```python
from build123d import *

# Parameters (mm, degrees)
F1_DEPTH = 10
F2_R     = 3.5
F3_SIZE  = 1
F4_R     = 1


# Not quite as in the source:
# - a feature names something its author has since deleted; it is built from what else it names


with BuildPart() as f1:
    # F0 (on Top) → F1 (new body)
    with BuildSketch(Plane.XY):
        with BuildLine():
            ThreePointArc((-44.3848475016, -14.7620242305), (-53.4374201274, 3.0310367894), (-39.6333784075, 17.4529133594))
            Line((-39.6333784075, 17.4529133594), (-39.6333784075, 67.7640176489))
            ThreePointArc((-39.6333784075, 67.7640176489), (-36.3720424684, 71.025353588), (-33.1107065292, 67.7640176489))
            Line((-33.1107065292, 67.7640176489), (-33.1107065292, 17.4529133594))
            ThreePointArc((-33.1107065292, 17.4529133594), (-19.3066648093, 3.0310367894), (-28.3592374351, -14.7620242305))
            Line((-28.3592374351, -14.7620242305), (-22.5229276093, -20.2994880054))
            ThreePointArc((-22.5229276093, -20.2994880054), (-11.4323530197, 2.249497469), (-25.5391483675, 23.0450718941))
            Line((-25.5391483675, 23.0450718941), (-25.5391483675, 67.7640176489))
            ThreePointArc((-25.5391483675, 67.7640176489), (-36.3720424684, 78.5969117497), (-47.2049365692, 67.7640176489))
            Line((-47.2049365692, 67.7640176489), (-47.2049365692, 23.0450718941))
            ThreePointArc((-47.2049365692, 23.0450718941), (-61.311731917, 2.249497469), (-50.2211573274, -20.2994880054))
            Line((-50.2211573274, -20.2994880054), (-44.3848475016, -14.7620242305))
        make_face()
    extrude(amount=F1_DEPTH)

    # F2
    f2_edges = [f1.edges().sort_by_distance(p)[0] for p in [
        (-50.221157, -20.299488, 5),
        (-44.384848, -14.762024, 5),
        (-28.359237, -14.762024, 5),
        (-22.522928, -20.299488, 5),
    ]]
    fillet(f2_edges, radius=F2_R)

    # F3
    f3_edges = [f1.edges().sort_by_distance(p)[0] for p in [
        (-53.038502, 4.962794, 10),
        (-61.149218, 3.844419, 10),
        (-47.204937, 45.404545, 10),
        (-39.633378, 42.608466, 10),
        (-36.372042, 78.596912, 10),
        (-36.372042, 71.025354, 10),
        (-33.110707, 42.608466, 10),
        (-25.539148, 45.404545, 10),
        (-19.705582, 4.962794, 10),
        (-11.594867, 3.844419, 0),
        (-25.539148, 45.404545, 0),
        (-39.633378, 42.608466, 0),
        (-53.038502, 4.962794, 0),
    ]]
    chamfer(f3_edges, length=F3_SIZE)

    # F4
    f4_edges = [f1.edges().sort_by_distance(p)[0] for p in [
        (-39.633378, 17.452913, 5),
        (-33.110707, 17.452913, 5),
    ]]
    fillet(f4_edges, radius=F4_R)


solid = f1.part
```
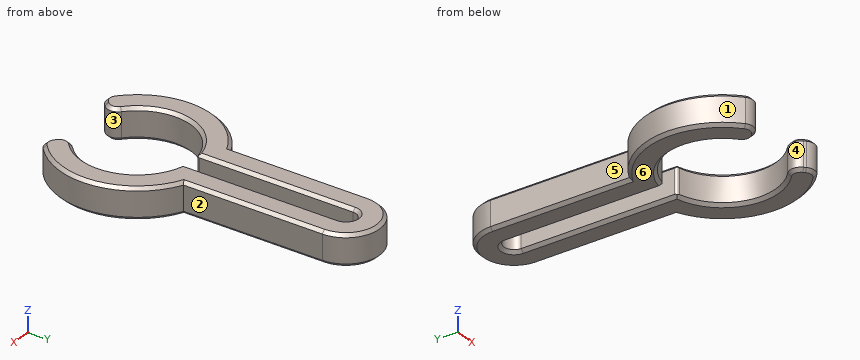
Could you check a few things on this model? Use its own coordinates, in mm. Face numbers are marked on the shaded views. A direction names the side the tool comes from. Give positions to 0.01 mm unless a question says otherwise; leave off trailing zeros. Loops run counter-clockwise (first coordinate to the right, second up) from the corner with the lowest first, then second, coordinate; pieces in that order, holes last. Notation, with made-up numbers: (79.25, 7) - (125.25, 7) arc R11 ccw to (125.25, 18) - close; hole circle Ø10 at (43, -2.75). An arc over 180 degrees is marked (long way). Answer in a Markdown table with one row per item. Add a question column.
Q1. Which directions (+Z, -Z, +X, -X, +Y, -Y) give clear straight access to the entire face, cutting with the end or side of a thin tool? Please do the marked faces 1, 2 and 3.
Q2. For pin 1 (6 mm diameter, centred on y = 4.5, z = 5.5, fed in from +X); pin 2 (4 mm diameter, centred on y = 54, z = 6.5, fed in from -X); pin 3 (4 mm diameter, centred on y = 50.5, z = 6, fed in from +X), each with a flat end and sliding along its axis, tell me the tip position at first contact or that it passes through.
Q3. Please list where these lines run through material, in increasing order: L1, parallel to X at y = 52, z = 7; L2, parallel to Y at x = -51, z = 4.75; L3, parallel to Y at x = -50.5, z = 2.25. Write a range as from..to.
Q4. We'd pull the mould along X, two halves only. Please class the marked faces 4, 5 and 6: +X half, -X half, draft (parallel to the pull), parting line (faces both ways), or undercut.
Q5. If we section it at A-A (y = 28): List the corners of the cut face in (x, z) for me, plus the area to 3 significant figures.
Q6. If we section it at B-B (z = 6.75): List the corners of the cut face in (x, y) for me.
The answers:
| question | item | result |
|---|---|---|
| 1 | face 1 | +Z, -Z, -X |
| 1 | face 2 | +Z, -Z, +X, +Y |
| 1 | face 3 | +Z, -Z |
| 2 | pin 1 | stops at x = -11.39 |
| 2 | pin 2 | stops at x = -47.2 |
| 2 | pin 3 | stops at x = -25.54 |
| 3 | L1 | x = -47.2..-39.63, -33.11..-25.54 |
| 3 | L2 | y = -19.18..-8.63, 9.66..20.79 |
| 3 | L3 | y = -19.21..-9.38, 10.41..21.14 |
| 4 | face 4 | undercut |
| 4 | face 5 | -X half |
| 4 | face 6 | draft |
| 5 | outline | (-47.2, 1) - (-46.2, 0) - (-40.63, 0) - (-39.63, 1) - (-39.63, 9) - (-40.63, 10) - (-46.2, 10) - (-47.2, 9) - close; (-33.11, 1) - (-32.11, 0) - (-26.54, 0) - (-25.54, 1) - (-25.54, 9) - (-26.54, 10) - (-32.11, 10) - (-33.11, 9) - close |
| 5 | area | 147 mm^2 |
| 6 | outline | (-52.77, -18.36) arc R3.5 ccw to (-48.07, -18.25) - (-47.52, -17.74) arc R3.5 ccw to (-47.64, -12.55) arc R17.25 cw to (-40.4, 17.29) arc R1 ccw to (-39.63, 18.26) - (-39.63, 67.76) arc R3.26 cw to (-33.11, 67.76) - (-33.11, 18.26) arc R1 ccw to (-32.34, 17.29) arc R17.25 cw to (-25.1, -12.55) arc R3.5 ccw to (-25.23, -17.74) - (-24.68, -18.25) arc R3.5 ccw to (-19.97, -18.36) arc R25 ccw to (-25.54, 23.05) - (-25.54, 67.76) arc R10.83 ccw to (-47.2, 67.76) - (-47.2, 23.05) arc R25 ccw to start |
